Read the model definition and answer for the solid it produces. Units are mm, in the model's axes. Face numbers are marked on the shaded views. A direction names the side the tool comes from. Give positions to 0.01 mm unless a question says otherwise; leave off trailing zeros. Loops run counter-clockwise (first coordinate to the right, second up) from the corner with the lowest first, then second, coordinate; pieces in that order, holes last. Notation, with made-up numbers: (5.25, -5) - (63.25, -5) arc R20 ccw to (63.25, 20) - close; hole circle Ø9 at (85, 15). An arc over 180 degrees is marked (long way). Write each question's results on one line, items separated by ' | '. Start each with the question number.
Q1. Determine the mould class of the marked faces 3, 4 and 5 for opening direction Z: +Z half, -Z half, draft (parallel to the pull), parting line (faces both ways), or undercut.
Q2. For the marked faces 1 and 2, determine the directions among +Z, -Z, +X, -X, +Y, -Y from which every point of the face is accessible in a straight line to the end or side of a thin tool.
Q3. The part is cut by section D-D, the plane y = -18. Write down the section's boundary in (x, z) (3 decimals), plus the area to 3 significant figures.
Q4. The part is cut by section C-C, the plane z = 16.75. Write down the section's boundary in (x, y).
Q5. The part is cut by section B-B, the plane y = 10. Write down the section's boundary in (x, z) (3 decimals), plus the area to 3 significant figures.
Q6. Find the intervals of material crossed by line 1 (Z direction, x = 52, y = -9) (3 decimals); line 2 (X direction, y = -21, z = 9); line 3 (Z direction, x = 42, y = 7) (3 decimals), in increasing order. Write a range as from..to.
Q7. Given pin 1 (1.5 mm diameter, centred on y = 3.5, z = 19, fed in from -X); pin 2 (3 mm diameter, centred on y = 9.5, z = 15, fed in from +X); pin 3 (9 mm diameter, centred on x = -44.5, y = 10, fed in from +Z) (3 decimals); pin 4 (2.5 mm diameter, centred on x = 47.625, y = -25.4, fed in from -Z), each flat-ended and moving along its own axis, determine where each tip first touches the part or whether it passes through.
Q8. The part is cut by section A-A, the plane y = 25.4. Write down the section's boundary in (x, z) (3 decimals).
```python
from build123d import *

# Parameters (mm, degrees)
SKETCH1_W           = 78
SKETCH1_H           = 70
BOSS_EXTRUDE1_DEPTH = 28.575
SKETCH2_W           = 115
SKETCH2_H           = 70
BOSS_EXTRUDE2_DEPTH = 3.175
SKETCH3_R           = 2
CUT_EXTRUDE1_DEPTH  = 74.128521283
SKETCH4_R           = 5
BOSS_EXTRUDE3_DEPTH = 10


with BuildPart() as part:
    # Sketch1 → Boss-Extrude1 (new body)
    with BuildSketch(Plane.XY):
        Rectangle(SKETCH1_W, SKETCH1_H)
    extrude(amount=BOSS_EXTRUDE1_DEPTH)

    # Sketch2 → Boss-Extrude2 (add)
    with BuildSketch(Plane(origin=(0, 0, 0), x_dir=(-1, 0, 0), z_dir=(0, 0, -1))):
        Rectangle(SKETCH2_W, SKETCH2_H)
    extrude(amount=-BOSS_EXTRUDE2_DEPTH)

    # Sketch3 → Cut-Extrude1 (cut, through all)
    with BuildSketch(Plane(origin=(0, 0, 0), x_dir=(-1, 0, 0), z_dir=(0, 0, -1))):
        with Locations((-47.625, 25.4)):
            Circle(SKETCH3_R)
        with Locations((47.625, 25.4)):
            Circle(SKETCH3_R)
        with Locations((47.625, -25.4)):
            Circle(SKETCH3_R)
        with Locations((-47.625, -25.4)):
            Circle(SKETCH3_R)
    extrude(amount=-CUT_EXTRUDE1_DEPTH, mode=Mode.SUBTRACT)

    # Sketch4 → Boss-Extrude3 (add)
    with BuildSketch(Plane.ZY.offset(-39)):
        with Locations(Location((13.575, 10, 0), (0, 0, 270))):
            Circle(SKETCH4_R)
    extrude(amount=-BOSS_EXTRUDE3_DEPTH)


solid = part.part
```
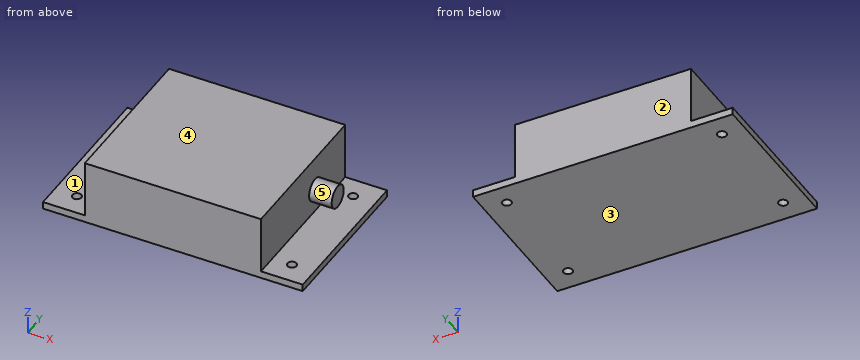
Check sheet entries:
1) face 3: -Z half | face 4: +Z half | face 5: undercut
2) face 1: +Z, -X, +Y, -Y | face 2: +Z, -Z, +X, -X, +Y
3) outline: (-57.5, 0) - (57.5, 0) - (57.5, 3.175) - (39, 3.175) - (39, 28.575) - (-39, 28.575) - (-39, 3.175) - (-57.5, 3.175) - close | area: 2,350 mm^2
4) outline: (-39, -35) - (39, -35) - (39, 6.14) - (49, 6.14) - (49, 13.86) - (39, 13.86) - (39, 35) - (-39, 35) - close
5) outline: (-57.5, 0) - (57.5, 0) - (57.5, 3.175) - (39, 3.175) - (39, 8.575) - (49, 8.575) - (49, 18.575) - (39, 18.575) - (39, 28.575) - (-39, 28.575) - (-39, 3.175) - (-57.5, 3.175) - close | area: 2,450 mm^2
6) line 1: z = 0..3.175 | line 2: x = -39..39 | line 3: z = 0..3.175, 9.575..17.575
7) pin 1: stops at x = -39 | pin 2: stops at x = 49 | pin 3: stops at z = 3.175 | pin 4: passes through
8) outline: (-57.5, 0) - (-49.625, 0) - (-49.625, 3.175) - (-57.5, 3.175) - close; (-45.625, 0) - (45.625, 0) - (45.625, 3.175) - (39, 3.175) - (39, 28.575) - (-39, 28.575) - (-39, 3.175) - (-45.625, 3.175) - close; (49.625, 0) - (57.5, 0) - (57.5, 3.175) - (49.625, 3.175) - close
